Here's how the part is built. I have some questions about the finished solid (model axes, mm). A direction names the side the tool comes from. Coordinates: 2 decimals unless noted, no trailing zeros. Write each loop counter-clockwise with the first axis right and the second up, starting at its lowest first coordinate (ties: lowest second). Pieces come first, ordered by that corner, then holes. Notation, with made-up numbers: (2, 22.25) -> (18, 22.25) arc R12 ccw to (18, 33.25) -> close; hole circle Ø6 at (-17.5, 38.5). An arc over 180 degrees is marked (long way). Put each result on its own line as item: value.
```python
from build123d import *

# Parameters (mm, degrees)
F1_DEPTH = 30.95
F2_DEPTH = 18
F4_DEPTH = 4
F5_DEPTH = 4
F6_D     = 5


with BuildPart() as f1:
    # F0 (on Top) → F1 (new body)
    with BuildSketch(Plane.XY):
        with BuildLine():
            ThreePointArc((31.4718047667, -14.9216086508), (33.9800813715, -7.6474159027), (34.83, 0))
            ThreePointArc((34.83, 0), (23.6128968094, 25.6039060354), (-2.8134110978, 34.7161866857))
            ThreePointArc((-2.8134110978, 34.7161866857), (-31.4718050367, 14.9216080814), (-28.6583943208, -19.7945784232))
            ThreePointArc((-28.6583943208, -19.7945784232), (2.8134104188, -34.7161867407), (31.4718047667, -14.9216086508))
        make_face()
        with BuildLine():
            ThreePointArc((8.6120840205, 29.5037664345), (24.589963678, 18.4383814722), (30.735, 0))
            ThreePointArc((30.735, 0), (24.589963678, -18.4383814722), (8.6120840205, -29.5037664345))
            ThreePointArc((8.6120840205, -29.5037664345), (6.8985351632, -29.9508002832), (5.1620840205, -30.2984011718))
            ThreePointArc((5.1620840205, -30.2984011718), (-1.2450816151, -30.7097703797), (-7.5979159795, -29.7810660952))
            ThreePointArc((-7.5979159795, -29.7810660952), (-9.3391355058, -29.2817481207), (-11.0479159795, -28.6807213562))
            ThreePointArc((-11.0479159795, -28.6807213562), (-30.735, 0), (-11.0479159795, 28.6807213562))
            ThreePointArc((-11.0479159795, 28.6807213562), (-9.3391355058, 29.2817481207), (-7.5979159795, 29.7810660952))
            ThreePointArc((-7.5979159795, 29.7810660952), (-1.2450816151, 30.7097703797), (5.1620840205, 30.2984011718))
            ThreePointArc((5.1620840205, 30.2984011718), (6.8985351632, 29.9508002832), (8.6120840205, 29.5037664345))
        make_face(mode=Mode.SUBTRACT)
    extrude(amount=F1_DEPTH)

    # F0 (on Top) → F2 (join)
    with BuildSketch(Plane.XY):
        with BuildLine():
            Line((8.6120840205, 28.6807213562), (8.6120840205, 29.5037664345))
            ThreePointArc((8.6120840205, 29.5037664345), (6.8985351632, 29.9508002832), (5.1620840205, 30.2984011718))
            Line((5.1620840205, 30.2984011718), (5.1620840205, 12.6006845385))
            Line((5.1620840205, 12.6006845385), (-7.5979159795, 12.6006845385))
            Line((-7.5979159795, 12.6006845385), (-7.5979159795, 29.7810660952))
            ThreePointArc((-7.5979159795, 29.7810660952), (-9.3391355058, 29.2817481207), (-11.0479159795, 28.6807213562))
            Line((-11.0479159795, 28.6807213562), (-11.0479159795, -28.6807213562))
            ThreePointArc((-11.0479159795, -28.6807213562), (-9.3391355058, -29.2817481207), (-7.5979159795, -29.7810660952))
            Line((-7.5979159795, -29.7810660952), (-7.5979159795, -22.835))
            Line((-7.5979159795, -22.835), (5.1620840205, -22.835))
            Line((5.1620840205, -22.835), (5.1620840205, -30.2984011718))
            ThreePointArc((5.1620840205, -30.2984011718), (6.8985351632, -29.9508002832), (8.6120840205, -29.5037664345))
            Line((8.6120840205, -29.5037664345), (8.6120840205, 28.6807213562))
        make_face()
        Polygon((5.1620840205, -17.415), (-7.5979159795, -17.415), (-7.5979159795, 5.935), (-4.9679159795, 5.935), (-4.9679159795, 8.565), (2.5320840205, 8.565), (2.5320840205, 5.935), (5.1620840205, 5.935), align=None, mode=Mode.SUBTRACT)
    extrude(amount=F2_DEPTH)

    # F0 (on Top) → F4 (join)
    with BuildSketch(Plane.XY):
        with BuildLine():
            ThreePointArc((-28.6583943208, -19.7945784232), (-31.4718050367, 14.9216080814), (-2.8134110978, 34.7161866857))
            Line((-2.8134110978, 34.7161866857), (-28.4157888205, 32.6413624978))
            ThreePointArc((-28.4157888205, 32.6413624978), (-44.8719442624, 21.2749669357), (-43.2564346771, 1.3403204934))
            Line((-43.2564346771, 1.3403204934), (-28.6583943208, -19.7945784232))
        make_face()
        with BuildLine():
            ThreePointArc((-2.8134110978, 34.7161866857), (23.6128968094, 25.6039060354), (34.83, 0))
            ThreePointArc((34.83, 0), (33.9800813715, -7.6474159027), (31.4718047667, -14.9216086508))
            Line((31.4718047667, -14.9216086508), (42.4761435474, 8.2881137382))
            ThreePointArc((42.4761435474, 8.2881137382), (40.8606339622, 28.2227601805), (22.7889689351, 36.7910110608))
            Line((22.7889689351, 36.7910110608), (-2.8134110978, 34.7161866857))
        make_face()
    extrude(amount=F4_DEPTH)

    # F0 (on Top) → F5 (join)
    with BuildSketch(Plane.XY):
        with BuildLine():
            Line((20.467465742, -38.1313315542), (31.4718047667, -14.9216086508))
            ThreePointArc((31.4718047667, -14.9216086508), (2.8134104188, -34.7161867407), (-28.6583943208, -19.7945784232))
            Line((-28.6583943208, -19.7945784232), (-14.060354727, -40.929476236))
            ThreePointArc((-14.060354727, -40.929476236), (4.0113103002, -49.4977271163), (20.467465742, -38.1313315542))
        make_face()
    extrude(amount=F5_DEPTH)

    # F6 (through all)
    with Locations(Plane(origin=(0, 0, 0), x_dir=(1, 0, 0), z_dir=(0, 0, -1))):
        with Locations((-37.4550744891, -19.1883724183), (33.4754809737, -26.3264067471), (3.0176348519, 42.3848293722)):
            Hole(F6_D / 2)


solid = f1.part
```
Item 1: Imagine slicing it at C-C on z = 15. Write out the boundary of the cut face in (x, y) (3 decimals).
Output:
outline: circle Ø69.66 at (0, 0); hole (-11.048, -28.681) -> (-11.048, 28.681) arc R30.735 ccw to start; hole (-7.598, -29.781) arc R30.735 ccw to (5.162, -30.298) -> (5.162, -22.835) -> (-7.598, -22.835) -> close; hole (-7.598, -17.415) -> (5.162, -17.415) -> (5.162, 5.935) -> (2.532, 5.935) -> (2.532, 8.565) -> (-4.968, 8.565) -> (-4.968, 5.935) -> (-7.598, 5.935) -> close; hole (-7.598, 12.601) -> (5.162, 12.601) -> (5.162, 30.298) arc R30.735 ccw to (-7.598, 29.781) -> close; hole (8.612, -29.504) arc R30.735 ccw to (8.612, 29.504) -> close
Item 2: Imagine slicing it at B-B on x = -22. Write out the boundary of the cut face in (y, z).
Output:
outline: (-29.43, 0) -> (-21.46, 0) -> (-21.46, 30.95) -> (-27, 30.95) -> (-27, 4) -> (-29.43, 4) -> close; (21.46, 0) -> (33.16, 0) -> (33.16, 4) -> (27, 4) -> (27, 30.95) -> (21.46, 30.95) -> close
Item 3: For P1, Ø2, axis at y = 8, z = 6, coming from the +X side; P2, Ø3.5, axis at y = -28, z = 11.5, coming from the -X side; P3, Ø6.5, axis at x = -1, z = 6.5, coming from the +Y side; P4, Ø17.5, axis at x = -12, y = -40, coming from the +Z side, each with a flat end and sliding along its axis, tell me the tip position at first contact or that it passes through.
Output:
P1: stops at x = 34.12
P2: stops at x = -22.89
P3: stops at y = 35.03
P4: stops at z = 30.95
Item 4: If we mould it in two halves opening along Y, with no side actions, what happens to faces 3 (the flat face through (-1, -17.415, 9)), 4 (the cylindrical face through (3.56, -39.944, 2.028)), 5 (the cylindrical face through (3.72, -49.52, 1.97)), 6 (the cylindrical face through (-44.744, 21.539, 1.972))? For each: released by +Y, released by -Y, zero draft, split by the parting line, or undercut.
Output:
face 3: undercut
face 4: undercut
face 5: released by -Y
face 6: split by the parting line
Item 5: Imagine slicing it at D-D on y = -26.5. Write out the boundary of the cut face in (x, z), then the cut area to 3 significant figures.
Output:
outline: (-24.03, 0) -> (-15.57, 0) -> (-15.57, 30.95) -> (-22.6, 30.95) -> (-22.6, 4) -> (-24.03, 4) -> close; (-11.05, 0) -> (-7.6, 0) -> (-7.6, 18) -> (-11.05, 18) -> close; (5.16, 0) -> (8.61, 0) -> (8.61, 18) -> (5.16, 18) -> close; (15.57, 0) -> (25.98, 0) -> (25.98, 4) -> (22.6, 4) -> (22.6, 30.95) -> (15.57, 30.95) -> close
area: 579 mm²
Item 6: Which directions (+Z, -Z, +X, -X, +Y, -Y) give clear straight access to the entire face, cutting with the end or side of a thin tool? Please do faces 1 (the flat face through (8, 4, 0)), 2 (the flat face through (-7.598, -6, 9)).
Output:
face 1: -Z, +X, -X, +Y, -Y
face 2: +Z, -Z
Item 7: Imagine slicing it at A-A on z = 27.5. Write out the boundary of the cut face in (x, y) (3 decimals).
Output:
outline: circle Ø69.66 at (0, 0); hole circle Ø61.47 at (0, 0)
Item 8: Please list where these lines run through material, in increasing order: line 1 along X through (y, z) = (-10.5, 11); line 2 along X through (y, z) = (-18.5, 6); line 3 along X through (y, z) = (5.5, 17). Write a range as from..to.
Output:
line 1: x = -33.21..-28.89, -11.05..-7.6, 5.16..8.61, 28.89..33.21
line 2: x = -29.51..-24.54, -11.05..8.61, 24.54..29.51
line 3: x = -34.39..-30.24, -11.05..-7.6, 5.16..8.61, 30.24..34.39
